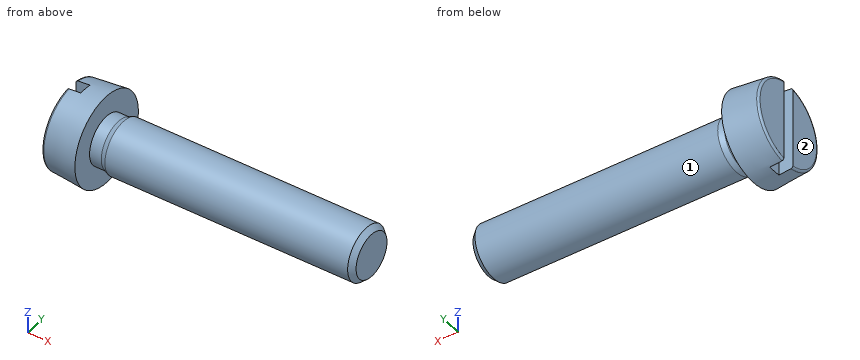
Autodesk Inventor part; units mm, degrees
ref_plane "Work Plane1" through (30.1625, 0, 0) normal (0, 0, -1) x (1, 0, 0)
ref_plane "YZ Plane" through (0, 0, 0) normal (1, 0, 0) x (0, 1, 0)
ref_plane "XZ Plane" through (0, 0, 0) normal (0, 1, 0) x (-1, 0, 0)
sketch "Sketch1" plane through (0, 0, 0) normal (0, 0, 1) x (1, 0, 0)
  line L0 (-3.3, 0) -> (25, 0)
  line L1 (25, 0) -> (25, 2.5)
  line L2 (25, 2.5) -> (1.6, 2.5)
  line L3 (1.6, 2.5) -> (1.1091, 2.2835)
  line L4 (1.1091, 2.2835) -> (0, 2.2835)
  line L5 (0, 2.2835) -> (0, 4.25)
  line L6 (-8.96, 0) -> (30.66, 0)
  line L7 (0, -0.85) -> (0, 5.1)
  line L8 (-3.3, 0) -> (-3.3, 3.9613)
  line L9 (0, 4.25) -> (-3.3, 3.9613)
  line L10 (1.6, 2.5) -> (0, 2.5) construction
  dimension "d0" = 25
  dimension "d1" = 23.4
  dimension "d2" = 0.4909
  dimension "d3" = 3.3
  dimension "d4" = 5
  dimension "d5" = 4.567
  dimension "d9" = 8.5
  dimension "d10" = 5
revolve "Body" add sketch "Sketch1" angle 360 about axis through (-3.3, 0, 0) along (1, 0, 0)
sketch "Sketch2" plane through (-3.3, 0, 0) normal (-1, 0, 0) x (0, 0, 1)
  circle A0 centre (0, 0) radius 4.25
  line L0 (0, 0) -> (0, 3.9613)
  line L1 (-4.25, 0.6) -> (4.25, 0.6)
  line L2 (4.25, 0.6) -> (4.25, -0.6)
  line L3 (4.25, -0.6) -> (-4.25, -0.6)
  line L4 (-4.25, -0.6) -> (-4.25, 0.6)
  line L5 (-4.25, 0) -> (4.25, 0) construction
  line L6 (0, 0.6) -> (0, -0.6) construction
  point P0 (0, 0)
  dimension "d11" = 1.2
  dimension "d12" = 8.5
fillet "Fillet1" radius 0.2 1 edges at (-3.3, -3.9613, 0)
extrude "Slot" cut sketch "Sketch2" against normal blind 1.3 contours A0 L3 L1 | L2 L3 A0 | A0 L1 L2 | A0 L4 L1 | L3 L4 A0
thread "Thread"
chamfer "Chamfer1" distance 0.433 distance2 0.4909 1 edges at (25, -2.5, 0) measured on face at (25, 0.6238, 0.5526)
ref_plane "Work Plane1" through (30.1625, 0, 0) normal (0, 0, -1) x (1, 0, 0)
equation "\"d11\" = SBR"
equation "\"d12\" = KOD"
equation "\"d14\" = RR"
equation "\"d19\" = STI"
equation "\"d15\" = GEL"
equation "\"d17\" = -0.5 * SPD + 0.5 * GD"
equation "\"d0\" = NLG"
equation "\"d1\" = GEL"
equation "\"d3\" = KOH"
equation "\"d4\" = GD"
equation "\"d5\" = BDM"
equation "\"d9\" = KOD"
equation "\"d10\" = KEWI"
equation "\"GD\" = 5"
equation "\"NLG\" = 25"
equation "\"GEL\" = 23.4"
equation "\"KOD\" = 8.5"
equation "\"KOH\" = 3.3"
equation "\"GAL\" = 0.61345 * PTC"
equation "\"SPD\" = 4.13397"
equation "\"BDM\" = 4.56699"
equation "\"GUL\" = 0.61345 * PTC"
equation "\"RR\" = 0.2"
equation "\"SBR\" = 1.2"
equation "\"STI\" = 1.3"
equation "\"KEWI\" = 5deg"
equation "\"PTC\" = 0.8"
equation "\"THREADDIA\" = 5"
equation "\"TOA\" = 30deg"
equation "\"NND\" = 5"
equation "\"GD1\" = THREADDIA - 1.2269 * PTC"
properties part number "DIN 84 - M5 x 25" material "Steel, Mild"
Verification items for the finished model (mm, model axes). Face numbers are marked on the shaded views. A direction names the side the tool comes from. Give positions to 0.01 mm unless a question says otherwise; leave off trailing zeros. Order: outer loops, then holes, each group sorted by start corner. A loop starts at its lowest first (then second) coordinate and runs counter-clockwise, first axis right, second up. Notation, with made-up numbers: M 44,44 L 67,44 A32 ccw 67,78 Z; hole C -36,82 d1. An arc over 180 degrees is marked long. Answer in a Markdown table with one row per item. Add a question column.
Item 1: Section check C-C, the plane x = 12.5. Enter the section's corners in (y, z).
Item 2: Gauge pin test, flat ends, axial feed: pin 1 (4 mm diameter, centred on x = 11, y = 2, fed in from +Z); pin 2 (1 mm diameter, centred on x = -2.5, z = -0.5, fed in from -Y); pin 3 (1 mm diameter, centred on x = 9, z = -1.5, fed in from -Y). Record the tip position at first contact, or that the pin passes through.
Item 3: Tool access check on the marked faces 1 and 2. Record the directions out of +Z, -Z, +X, -X, +Y, -Y that give a thin tool (end or side, any length) a straight path to the whole face; none if there is none.
Item 4: Section check A-A, the plane y = 0. Enter the section's corners in (x, z).
Item 5: Section check B-B, the plane z = 0. Enter the section's corners in (x, y).
Item 6: Scan lines: probe 1 along X at (y, z) = (1.75, 3); probe 2 along X at (y, z) = (-0.5, 3); probe 3 along Y at (x, z) = (18.75, -0.75). Record each from-to range of solid material in increasing order. Write a range as from..to.
Filled sheet:
| question | item | result |
|---|---|---|
| 1 | outline | C 0,0 d5 |
| 2 | pin 1 | stops at z = 2.5 |
| 2 | pin 2 | stops at y = -4.06 |
| 2 | pin 3 | stops at y = -2.29 |
| 3 | face 1 | +X |
| 3 | face 2 | +Z, -Z, -X, +Y, -Y |
| 4 | outline | M -2,-4.08 L 0,-4.25 L 0,-2.28 L 1.11,-2.28 L 1.6,-2.5 L 24.51,-2.5 L 25,-2.07 L 25,2.07 L 24.51,2.5 L 1.6,2.5 L 1.11,2.28 L 0,2.28 L 0,4.25 L -2,4.08 Z |
| 5 | outline | M -3.3,-3.78 A0.2 ccw -3.12,-3.98 L 0,-4.25 L 0,-2.28 L 1.11,-2.28 L 1.6,-2.5 L 24.51,-2.5 L 25,-2.07 L 25,2.07 L 24.51,2.5 L 1.6,2.5 L 1.11,2.28 L 0,2.28 L 0,4.25 L -3.12,3.98 A0.2 ccw -3.3,3.78 L -3.3,0.6 L -2,0.6 L -2,-0.6 L -3.3,-0.6 Z |
| 6 | probe 1 | x = -3.3..0 |
| 6 | probe 2 | x = -2..0 |
| 6 | probe 3 | y = -2.38..2.38 |
